Could you check a few things on this model? Use its own coordinates, in mm. A direction names the side the tool comes from. Coordinates: 2 decimals unless noted, no trailing zeros. Order: outer loops, then holes, each group sorted by start corner. A loop starts at its lowest first (then second) coordinate and runs counter-clockwise, first axis right, second up. Notation, with made-up numbers: (40.5, -34.75) - (71.5, -34.75) arc R12 ccw to (71.5, -22.75) - close; hole circle Ø11 at (-30, 38.5). An arc over 180 degrees is marked (long way). Answer as a JSON object with one key per item and string values. Group by question number.
(1) Which directions (+Z, -Z, +X, -X, +Y, -Y) give clear straight access to the entire face, cutting with the end or side of a thin tool? Please do faces 5 (the cylindrical face through (7.14, -24.21, -35.47)), 6 (the flat face through (31.946, -13, -9)).
(2) Imagine slicing it at A-A, the plane y = -12.5. Write out the boundary of the cut face in (x, z), and give its area (3 significant figures).
(3) Please list where these lines run through material, in increasing order: probe 1 along X at (y, z) = (-18, -29); probe 2 along X at (y, z) = (-20.5, -40); probe 3 along Z at (x, y) = (-11, -23.25).
(4) Will these pins go through, and if not, where does the flat tip stop? P1, Ø4, axis at x = 5.5, y = -21, coming from the -Z side; P2, Ø1, axis at x = 21, y = -15.5, coming from the +Z side; P3, Ø6, axis at x = 6.48, y = -19.17, coming from the +Z side; P4, Ø8, axis at x = -2, z = -15.5, coming from the +Y side.
(5) We'd pull the mould along X, two halves only. Please class faces 1 (the conical face through (7.32, -19.44, -20.43)), 2 (the flat face through (-18.995, -13, -9)), 3 (the cylindrical face through (7.04, -12.52, 57.41)), 4 (the flat face through (6, -25.4, 5)): pulls with the +X half, pulls with the -X half, needs draft (parallel to the pull), parting line crosses it, or undercut.
(6) Imagine slicing it at B-B, the plane x = -6.5. Write out the boundary of the cut face in (y, z), and give its area (3 significant figures).
from build123d import *

# Parameters (mm, degrees)
F0_W     = 50.9416162968
F0_H     = 80.2978053689
F1_DEPTH = 25.4
F3_D     = 10.16
F3_DEPTH = 25.4
F3_TIP   = 3.0523719447


with BuildPart() as f1:
    # F0 (on Front) → F1 (new body)
    with BuildSketch(Plane.XZ):
        with BuildLine():
            ThreePointArc((31.9464355707, 31.946439296), (6.4756274223, 57.4172474444), (-18.9951807261, 31.946439296))
            Line((-18.9951807261, 31.946439296), (31.9464355707, 31.946439296))
        make_face()
        with Locations((6.4756274223, -8.2024633884)):
            Rectangle(F0_W, F0_H)
    extrude(amount=F1_DEPTH)

    # F3
    with Locations(Plane(origin=(0, 0, -48.3513660729), x_dir=(1, 0, 0), z_dir=(0, 0, -1))):
        with Locations((6.4756274223, 19.1739164293)):
            Hole(F3_D / 2, depth=F3_DEPTH)
            with Locations((0, 0, -(F3_DEPTH + F3_TIP / 2))):  # 118° drill point
                Cone(0, F3_D / 2, F3_TIP, mode=Mode.SUBTRACT)


solid = f1.part
Result set:
{
 "1": {"face 5": "-Z", "face 6": "+Z, -Z, +X, +Y, -Y"},
 "2": {"outline": "(-19, -48.35) - (31.95, -48.35) - (31.95, 31.95) arc R25.47 ccw to (-19, 31.95) - close", "area": "5,110 mm^2"},
 "3": {"probe 1": "x = -19 to 1.53, 11.42 to 31.95", "probe 2": "x = -19 to 1.57, 11.38 to 31.95", "probe 3": "z = -48.35 to 50.48"},
 "4": {"P1": "stops at z = -22.34", "P2": "stops at z = 53.21", "P3": "stops at z = 57.42", "P4": "stops at y = 0"},
 "5": {"face 1": "undercut", "face 2": "pulls with the -X half", "face 3": "parting line crosses it", "face 4": "needs draft"},
 "6": {"outline": "(-25.4, -48.35) - (0, -48.35) - (0, 53.86) - (-25.4, 53.86) - close", "area": "2,600 mm^2"}
}
